Design review of the part built by this model. Coordinates are the model's own, in mm. A direction names the side the tool comes from. Coordinates: 2 decimals unless noted, no trailing zeros. Write each loop counter-clockwise with the first axis right and the second up, starting at its lowest first coordinate (ties: lowest second). Pieces come first, ordered by that corner, then holes. Notation, with made-up numbers: (59, -10.75) - (111, -10.75) arc R24 ccw to (111, 3.25) - close; hole circle Ø5 at (26.5, -6.5). An arc over 180 degrees is marked (long way). Answer as CSV lines item,"result". Start each with the question number.
Q1. For line 1 along Y through (x, z) = (0, 0.1); line 2 along Z through (x, y) = (18.25, 4); line 3 along Z through (x, y) = (10, 2.25), list the stretches that pass through material, from the lowest coordinate up. Write a range as [from, to].
Q2. We need section B-B (y = 1). State how many separate pieces and enclosed holes the cut face has, plus the area to 3 significant figures.
Q3. Clearance check with flat-ended pins moving along their axes: pin 1 (4 mm diameter, centred on x = 2, z = 15.5, fed in from +Y); pin 2 (3 mm diameter, centred on x = 6.5, y = -0.5, fed in from +Z); pin 3 (3.5 mm diameter, centred on x = 0, y = 0, fed in from +Z); pin 4 (4 mm diameter, centred on x = 10, z = 30, fed in from -Y). State where each tip first meets the part, or that it passes through.
Q4. Mouldability with a two-part tool opening along X and no side actions: class faces 1 (the face through (15, 1, 16)), 2 (the face through (10, -5, 1)), 3 (the face through (5, 1, 16)), 4 (the face through (16.66, -1.05, 1.77)) as pulls with the +X half, pulls with the -X half, needs draft (parallel to the pull), parting line crosses it, or undercut.
Q5. Machinability: for faces 5 (the face through (-3.233, 1.341, 1.768)), 6 (the face through (7, 1, 34)), 7 (the face through (10, -3, 4)), 8 (the face through (-5, 0, 1)), 9 (the face through (10, 3, 19)), which of the approach directions +Z, -Z, +X, -X, +Y, -Y give a long, thin tool a straight path to every point of the face, cutting with its end or side? Answer none if there is none.
Q6. We need section A-A (y = -1). Write out the cut boundary in (x, z), plus the area to 3 significant figures.
Q7. We need section C-C (z = 24). Write out the cut boundary in (x, y), plus the area to 3 significant figures.
Q8. We need section D-D (x = 3). Write out the cut boundary in (y, z), plus the area to 3 significant figures.
Autodesk Fusion 360 part; units mm, degrees
sketch "Sketch1" plane through (0, 0, 0) normal (0, 0, 1) x (1, 0, 0)
  line L0 (0, -5) -> (20, -5)
  arc A0 (20, -5) -> (20, 5) centre (20, 0) ccw
  line L1 (20, 5) -> (0, 5)
  arc A1 (0, 5) -> (0, -5) centre (0, 0) ccw
  line L2 (0, 0) -> (20, 0) construction
  dimension "d1" = 10
extrude "Extrude1" add sketch "Sketch1" along normal blind 3
sketch "Sketch2" plane through (0, 0, 3) normal (0, 0, 1) x (-1, 0, 0)
  arc A0 (0, -5) -> (0, 5) centre (0, 0) ccw
  line L0 (0, 5) -> (-20, 5)
  arc A1 (-20, 5) -> (-20, -5) centre (-20, 0) ccw
  line L1 (-20, -5) -> (0, -5)
  circle A2 centre (0, 0) radius 3.5
  circle A3 centre (-20, 0) radius 3.5
  dimension "d4" = 7
extrude "Extrude2" cut sketch "Sketch2" against normal blind 2.5 contours A2 | A3
sketch "Sketch3" plane through (0, 0, 0.5) normal (0, 0, 1) x (-1, 0, 0)
  circle A0 centre (0, 0) radius 3.5
  circle A1 centre (0, 0) radius 1.5
  circle A2 centre (-20, 0) radius 1.5
  dimension "d7" = 3
extrude "Extrude3" cut sketch "Sketch3" against normal blind 2 contours A1 | A2
sketch "Sketch4" plane through (0, 0, 3) normal (0, 0, 1) x (-1, 0, 0)
  circle A0 centre (0, 0) radius 3.5
  circle A1 centre (-20, 0) radius 3.5
  arc A2 (0, -5) -> (0, 5) centre (0, 0) ccw
  line L0 (0, 5) -> (-20, 5)
  arc A3 (-20, 5) -> (-20, -5) centre (-20, 0) ccw
  line L1 (-20, -5) -> (0, -5)
  line L2 (-15, -3) -> (-5, -3)
  line L3 (-5, -3) -> (-5, 3)
  line L4 (-5, 3) -> (-15, 3)
  line L5 (-15, 3) -> (-15, -3)
  line L6 (-15, -3) -> (-5, 3) construction
  line L7 (-5, -3) -> (-15, 3) construction
  point P0 (-10, 0)
extrude "Extrude4" add sketch "Sketch4" along normal blind 32 contours L2 L3 L4 L5
sketch "Sketch5" plane through (0, -3, 0) normal (0, -1, 0) x (1, 0, 0)
  line L0 (5, 3) -> (15, 3)
  line L1 (15, 3) -> (15, 35)
  line L2 (15, 35) -> (5, 35)
  line L3 (5, 35) -> (5, 3)
  line L4 (5, 35) -> (15, 35)
  line L5 (15, 35) -> (15, 25)
  line L6 (15, 25) -> (5, 25)
  line L7 (5, 25) -> (5, 35)
  dimension "d12" = 10
  dimension "d13" = 10
extrude "Extrude5" cut sketch "Sketch5" against normal blind 3 contours L1 L2 L3 L4 L5 L6 L7
sketch "Sketch6" plane through (0, 0, 0) normal (0, -1, 0) x (1, 0, 0)
  line L0 (5, 25) -> (15, 25)
  line L1 (15, 25) -> (15, 35)
  line L2 (15, 35) -> (5, 35)
  line L3 (5, 35) -> (5, 25)
  circle A0 centre (10, 30) radius 1.75
  dimension "d16" = 3.5
extrude "Extrude6" cut sketch "Sketch6" against normal blind 3 contours A0
fillet "Fillet1" radius 5 2 edges at (15, 1.5, 35) (5, 1.5, 35)
sketch "Sketch8" plane through (0, 0, 25) normal (0, 0, 1) x (-1, 0, 0)
  line L0 (-5, 3) -> (-15, 3)
  line L1 (-15, 3) -> (-15, 0)
  line L2 (-15, 0) -> (-5, 0)
  line L3 (-5, 0) -> (-5, 3)
  line L4 (-5, 0) -> (-15, 0)
  line L5 (-15, 0) -> (-15, 3)
  line L6 (-15, 3) -> (-5, 3)
  line L7 (-5, 3) -> (-5, 0)
extrude "Extrude7" cut sketch "Sketch8" against normal blind 20
Results list:
1,line 1,"y = [-5, -1.5], [1.5, 5]"
1,line 2,"z = [0, 3]"
1,line 3,"z = [0, 28.25], [31.75, 35]"
2,separate pieces,"3"
2,enclosed holes,"1"
2,area,"353 mm2"
3,pin 1,"passes through"
3,pin 2,"stops at z = 34.54"
3,pin 3,"stops at z = 0.5"
3,pin 4,"stops at y = 0"
4,face 1,"pulls with the +X half"
4,face 2,"needs draft"
4,face 3,"pulls with the -X half"
4,face 4,"undercut"
5,face 5,"+Z"
5,face 6,"+Z, -X, +Y, -Y"
5,face 7,"+Z, +X, -X, -Y"
5,face 8,"+Z, -Z, -X"
5,face 9,"+Z, +X, -X, +Y"
6,outline,"(-4.9, 0) - (-1.12, 0) - (-1.12, 0.5) - (-3.35, 0.5) - (-3.35, 3) - (-4.9, 3) - close; (1.12, 0) - (18.88, 0) - (18.88, 0.5) - (16.65, 0.5) - (16.65, 3) - (15, 3) - (15, 5) - (5, 5) - (5, 3) - (3.35, 3) - (3.35, 0.5) - (1.12, 0.5) - close; (21.12, 0) - (24.9, 0) - (24.9, 3) - (23.35, 3) - (23.35, 0.5) - (21.12, 0.5) - close"
6,area,"73.6 mm2"
7,outline,"(5, 0) - (15, 0) - (15, 3) - (5, 3) - close"
7,area,"30.0 mm2"
8,outline,"(-5, 0) - (5, 0) - (5, 3) - (1.8, 3) - (1.8, 0.5) - (-1.8, 0.5) - (-1.8, 3) - (-5, 3) - close"
8,area,"21.0 mm2"
